from build123d import *

# Parameters (mm, degrees)
SKETCH1_W           = 7
SKETCH1_H           = 3
SKETCH1_W_2         = 17
SKETCH1_H_2         = 3.275
BOSS_EXTRUDE1_DEPTH = 15
BOSS_EXTRUDE2_START = 7
SKETCH2_W           = 7
SKETCH2_H           = 3.275
SKETCH2_R           = 12.575
BOSS_EXTRUDE2_DEPTH = 7
SKETCH3_R           = 12.575
BOSS_EXTRUDE3_DEPTH = 2
BOSS_EXTRUDE4_DEPTH = 22
SKETCH5_W           = 3.1
SKETCH5_H           = 3.1
CUT_EXTRUDE1_DEPTH  = 5.1
SKETCH7_R           = 1.5
BOSS_EXTRUDE5_DEPTH = 7
CUT_EXTRUDE2_START  = -20
CUT_EXTRUDE2_DEPTH  = 20


with BuildPart() as part:
    # Sketch1 → Boss-Extrude1 (new body)
    with BuildSketch(Plane.XY):
        with Locations((12, 20.325)):
            Rectangle(SKETCH1_W, SKETCH1_H)
        with Locations((0, 20.325)):
            Rectangle(SKETCH1_W_2, SKETCH1_H)
        with Locations((-12, 20.325)):
            Rectangle(SKETCH1_W, SKETCH1_H)
        with Locations((0, 17.1875)):
            Rectangle(SKETCH1_W_2, SKETCH1_H_2)
        with BuildLine():
            ThreePointArc((-15.5, 0), (0, 15.5), (15.5, 0))
            Line((15.5, 0), (15.5, 15.55))
            Line((15.5, 15.55), (8.5, 15.55))
            Line((8.5, 15.55), (-8.5, 15.55))
            Line((-8.5, 15.55), (-15.5, 15.55))
            Line((-15.5, 15.55), (-15.5, 0))
        make_face()
        with BuildLine():
            ThreePointArc((-12.575, 0), (0, 12.575), (12.575, 0))
            Line((12.575, 0), (15.5, 0))
            ThreePointArc((15.5, 0), (0, 15.5), (-15.5, 0))
            Line((-15.5, 0), (-12.575, 0))
        make_face()
        with BuildLine():
            Line((15.5, 0), (12.575, 0))
            ThreePointArc((12.575, 0), (0, -12.575), (-12.575, 0))
            Line((-12.575, 0), (-15.5, 0))
            ThreePointArc((-15.5, 0), (0, -15.5), (15.5, 0))
        make_face()
        with BuildLine():
            ThreePointArc((-12.575, 0), (0, 12.575), (12.575, 0))
            Line((12.575, 0), (15.5, 0))
            ThreePointArc((15.5, 0), (0, 15.5), (-15.5, 0))
            Line((-15.5, 0), (-12.575, 0))
        make_face()
        with BuildLine():
            Line((15.5, 0), (12.575, 0))
            ThreePointArc((12.575, 0), (0, -12.575), (-12.575, 0))
            Line((-12.575, 0), (-15.5, 0))
            ThreePointArc((-15.5, 0), (0, -15.5), (15.5, 0))
        make_face()
    extrude(amount=BOSS_EXTRUDE1_DEPTH)

    # Sketch2 → Boss-Extrude2 (add)
    # profile 1 of 3: a face of its own
    with BuildSketch(Plane(origin=(0, 0, 0), x_dir=(-1, 0, 0), z_dir=(0, 0, -1)).offset(BOSS_EXTRUDE2_START)):
        with Locations((-12, 17.1875)):
            Rectangle(SKETCH2_W, SKETCH2_H)
    # profile 2 of 3: a face of its own
    with BuildSketch(Plane(origin=(0, 0, 0), x_dir=(-1, 0, 0), z_dir=(0, 0, -1)).offset(BOSS_EXTRUDE2_START)):
        with BuildLine():
            Line((-15.5, 15.55), (-15.5, 0))
            ThreePointArc((-15.5, 0), (0, -15.5), (15.5, 0))
            Line((15.5, 0), (15.5, 15.55))
            Line((15.5, 15.55), (8.5, 15.55))
            Line((8.5, 15.55), (8.5, 18.825))
            Line((8.5, 18.825), (15.5, 18.825))
            Line((15.5, 18.825), (15.5, 21.825))
            Line((15.5, 21.825), (-15.5, 21.825))
            Line((-15.5, 21.825), (-15.5, 18.825))
            Line((-15.5, 18.825), (-8.5, 18.825))
            Line((-8.5, 18.825), (-8.5, 15.55))
            Line((-8.5, 15.55), (-15.5, 15.55))
        make_face()
        Circle(SKETCH2_R, mode=Mode.SUBTRACT)
    # profile 3 of 3: a face of its own
    with BuildSketch(Plane(origin=(0, 0, 0), x_dir=(-1, 0, 0), z_dir=(0, 0, -1)).offset(BOSS_EXTRUDE2_START)):
        with Locations((12, 17.1875)):
            Rectangle(SKETCH2_W, SKETCH2_H)
    extrude(amount=-BOSS_EXTRUDE2_DEPTH)

    # Sketch3 → Boss-Extrude3 (add)
    with BuildSketch(Plane(origin=(0, 0, -7), x_dir=(-1, 0, 0), z_dir=(0, 0, -1))):
        Circle(SKETCH3_R)
    extrude(amount=-BOSS_EXTRUDE3_DEPTH)

    # Sketch4 → Boss-Extrude4 (add)
    with BuildSketch(Plane(origin=(0, 0, -7), x_dir=(-1, 0, 0), z_dir=(0, 0, -1))):
        with BuildLine():
            Line((15.5, -10.099504938), (15.5, 0))
            ThreePointArc((15.5, 0), (0, -15.5), (-15.5, 0))
            Line((-15.5, 0), (-15.5, -10.099504938))
            ThreePointArc((-15.5, -10.099504938), (0, -18.5), (15.5, -10.099504938))
        make_face()
    extrude(amount=-BOSS_EXTRUDE4_DEPTH)

    # Sketch5 → Cut-Extrude1 (cut)
    with BuildSketch(Plane(origin=(0, 0, -7), x_dir=(-1, 0, 0), z_dir=(0, 0, -1))):
        with Locations((0, -16.95)):
            Rectangle(SKETCH5_W, SKETCH5_H)
    extrude(amount=-CUT_EXTRUDE1_DEPTH, mode=Mode.SUBTRACT)

    # Sketch7 → Boss-Extrude5 (add)
    with BuildSketch(Plane.XY.offset(-5)):
        with Locations((6.2875, 10.890269453)):
            Circle(SKETCH7_R)
        with Locations((6.2875, -10.890269453)):
            Circle(SKETCH7_R)
    extrude(amount=BOSS_EXTRUDE5_DEPTH)

    # Sketch6 → Cut-Extrude2 (cut)
    with BuildSketch(Plane.XY.offset(15).offset(CUT_EXTRUDE2_START)):
        with BuildLine():
            ThreePointArc((12.575, 0), (11.245882841, -5.626788082), (7.539493977, -10.064127164))
            Line((7.539493977, -10.064127164), (15.5, -10.064127164))
            Line((15.5, -10.064127164), (15.5, 10.064127164))
            Line((15.5, 10.064127164), (7.539493977, 10.064127164))
            ThreePointArc((7.539493977, 10.064127164), (11.245882841, 5.626788082), (12.575, 0))
        make_face()
    extrude(amount=CUT_EXTRUDE2_DEPTH, mode=Mode.SUBTRACT)


solid = part.part
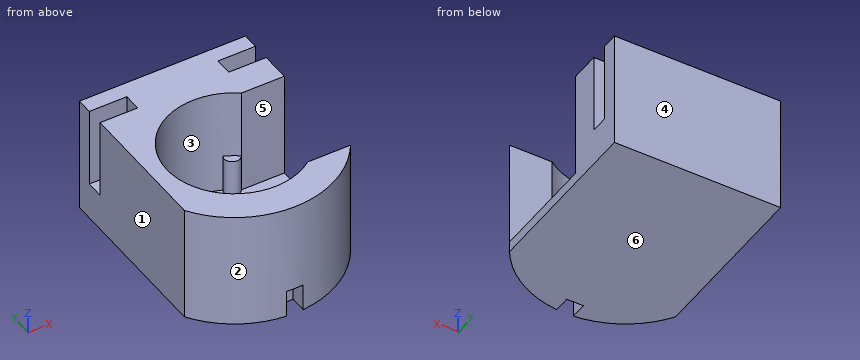
Verification items for the finished model (mm, model axes). Face numbers are marked on the shaded views. A direction names the side the tool comes from. Coordinates: 2 decimals unless noted, no trailing zeros. Order: outer loops, then holes, each group sorted by start corner. A loop starts at its lowest first (then second) coordinate and runs counter-clockwise, first axis right, second up. Notation, with made-up numbers: M 18,18.25 L 47,18.25 A18 cw 47,29.25 Z; hole C -24.5,15.5 d2. An arc over 180 degrees is marked long. Return JSON: item names as keys, results as strings.
1) Cross-section at B-B, the plane x = 0. Record the boundary of the cut face in (y, z) (3 decimals), and give its area (3 significant figures).
Answer list:
{"outline": "M -18.5,-1.9 L -15.4,-1.9 L -15.4,-7 L 21.825,-7 L 21.825,15 L 12.575,15 L 12.575,-5 L -12.575,-5 L -12.575,15 L -18.5,15 Z", "area": "368 mm2"}
2) Gauge pin test, flat ends, axial feed: pin 1 (1 mm diameter, centred on x = -10.5, y = 16.5, fed in from +Z); pin 2 (1.5 mm diameter, centred on y = -17.5, z = -4, fed in from +X); pin 3 (7.5 mm diameter, centred on x = 13.5, z = 6.5, fed in from -Y). Record the tip position at first contact, or that the pin passes through.
Answer list:
{"pin 1": "z = 0", "pin 2": "x = 7.85", "pin 3": "y = -15.72"}
3) Release check for a two-part mould opening along X. For the marked faces 1, 2, 3 and 4 record: +X half, -X half, draft (parallel to the pull), parting line (faces both ways), or undercut.
Answer list:
{"face 1": "-X half", "face 2": "parting line", "face 3": "undercut", "face 4": "draft"}
4) Thickness scan on L1, parallel to Y at x = 0, z = 2 (3 decimals); L2, parallel to Z at x = -9.5, y = -1.5; L3, parallel to Y at x = -7, z = 2.5 (3 decimals). Record the ranges inside material, lowest first. Write a range as [from, to].
Answer list:
{"L1": "[-18.5, -12.575], [12.575, 21.825]", "L2": "[-7, -5]", "L3": "[-17.125, -10.447], [10.447, 21.825]"}
5) Cross-section at A-A, the plane y = 17.5. Record the boundary of the cut face in (x, z).
Answer list:
{"outline": "M -15.5,-7 L 15.5,-7 L 15.5,0 L 8.5,0 L 8.5,15 L -8.5,15 L -8.5,0 L -15.5,0 Z"}
6) Access from +Z, -Z, +X, -X, +Y, -Y to the whole of each face (thin tool, end or side, straight path). Record for the marked faces 5 and 6.
Answer list:
{"face 5": "+Z, +X", "face 6": "-Z, +X, -X, +Y, -Y"}
7) Cross-section at D-D, the plane y = 0. Record the boundary of the cut face in (x, z) (3 decimals).
Answer list:
{"outline": "M -15.5,-7 L 15.5,-7 L 15.5,-5 L -12.575,-5 L -12.575,15 L -15.5,15 Z"}
